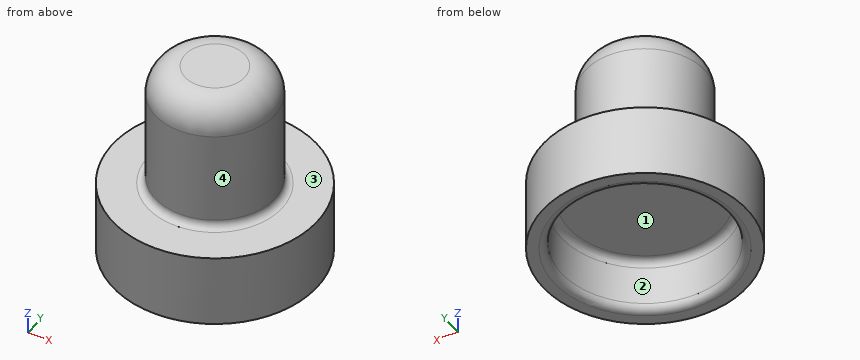
```python
from build123d import *

# Parameters (mm, degrees)
F2_R = 5.08
F3_R = 1.27
F4_R = 1.27


with BuildPart() as f1:
    # F0 (on Front) → F1 (revolve)
    with BuildSketch(Plane.XZ):
        Polygon((14.224, 0), (17.399, 0), (17.399, 12.394325), (10.16, 12.394325), (10.16, 34.484531), (0, 34.484531), (0, 9.219325), (14.224, 9.219325), align=None)
    revolve(axis=Axis((0, 0, 21.851928), (0, 0, 1)))

    # F2
    f2_edges = [f1.edges().sort_by_distance(p)[0] for p in [
        (-10.16, 0, 34.484531),
    ]]
    fillet(f2_edges, radius=F2_R)

    # F3
    f3_edges = [f1.edges().sort_by_distance(p)[0] for p in [
        (-10.16, 0, 12.394325),
    ]]
    fillet(f3_edges, radius=F3_R)

    # F4
    f4_edges = [f1.edges().sort_by_distance(p)[0] for p in [
        (-14.224, 0, 9.219325),
        (-14.224, 0, 0),
    ]]
    fillet(f4_edges, radius=F4_R)


solid = f1.part
```
Work out the finished part from the listing and answer in its coordinate system (mm). Face numbers are marked on the shaded views. Give positions to 0.01 mm unless a question says otherwise; leave off trailing zeros. Loops run counter-clockwise (first coordinate to the right, second up) from the corner with the lowest first, then second, coordinate; pieces in that order, holes last. Notation, with made-up numbers: (71, 88) -> (111, 88) arc R7 cw to (111, 97) -> close; hole circle Ø4 at (51.5, 75). An arc over 180 degrees is marked (long way). Write item = value, one per line. Start each with the question number.
(1) Given pin 1 Ø1.5 at (x, z) = (9.5, 22.5) entering from -Y; pin 2 Ø3 at (x, y) = (9, 2) entering from +Z; pin 3 Ø12 at (y, z) = (13, 22.5) entering from +X; pin 4 Ø12 at (x, z) = (-5.5, 9.5) entering from -Y, each flat-ended and moving along its own axis, determine where each tip first touches the part or whether it passes through.
(2) Find section A-A on z = 5. Give the vertices of the cut face in (x, y).
(3) Find the intervals of material crossed by probe 1 along Y at (x, z) = (0, 4.5); probe 2 along Z at (x, y) = (-2, -1.5); probe 3 along X at (y, z) = (-5.5, 3.5), in increasing order. Write a range as from..to.
(4) Find section B-B on z = 24. Give the vertices of the cut face in (x, y).
(5) The mould has two halves that part along Y. Classify the marked faces 1, 2, 3 and 4: +Y half, -Y half, draft (parallel to the pull), parting line (faces both ways), or undercut.
From the geometry:
q1.pin_1 = -5.16
q1.pin_2 = 33.74
q1.pin_3 = 7.36
q1.pin_4 = -17.4
q2.outline = circle Ø34.8 at (0, 0); hole circle Ø28.45 at (0, 0)
q3.probe_1 = -17.4..-14.22, 14.22..17.4
q3.probe_2 = 9.22..34.48
q3.probe_3 = -16.51..-13.12, 13.12..16.51
q4.outline = circle Ø20.32 at (0, 0)
q5.face_1 = undercut
q5.face_2 = undercut
q5.face_3 = draft
q5.face_4 = parting line
